```python
from build123d import *

# Parameters (mm, degrees)
BOSS_EXTRUDE1_DEPTH     = 12.5
SKETCH3_W               = 25
SKETCH3_H               = 11.5
CUT_EXTRUDE2_DEPTH      = 60.634302209
CUT_EXTRUDE1_DEPTH      = 60.634302209
CUT_EXTRUDE1_DEPTH_BACK = 60.634302209
SKETCH2_W               = 20.25
SKETCH2_H               = 8.5
SKETCH4_W               = 7.5
SKETCH4_H               = 20
CUT_EXTRUDE3_DEPTH      = 60.634302209
SKETCH8_R               = 2.55
PIN_HOLE_DEPTH          = 64.442887702
SKETCH9_R               = 3.5
COUNTERBORE_DEPTH       = 9
SKETCH7_R               = 2.55
CUT_EXTRUDE5_DEPTH      = 60.851900555
LPATTERN1_COUNT         = 2
LPATTERN1_PITCH         = 8.3
MIRROR2_COPY_1_SKETCH_R = 2.55
MIRROR2_COPY_1_DEPTH    = 60.851900555
FILLET1_R               = 5
CHAMFER1_SIZE           = 0.5
FILLET2_R               = 3


# Some blends are built 0.0001 mm under size
with BuildPart() as part:
    # Sketch1 → Boss-Extrude1 (new, symmetric)
    with BuildSketch(Plane.XY):
        Polygon((25, -30), (0, -30), (0, 30), (25, 30), (25, 0), (50, 0), (50, -30), align=None)
    extrude(amount=BOSS_EXTRUDE1_DEPTH, both=True)

    # Sketch3 → Cut-Extrude2 (cut, through all)
    with BuildSketch(Plane(origin=(0, 0, 0), x_dir=(1, 0, 0), z_dir=(0, 1, 0))):
        with Locations((37.5, -6.75)):
            Rectangle(SKETCH3_W, SKETCH3_H)
    extrude(amount=-CUT_EXTRUDE2_DEPTH, mode=Mode.SUBTRACT)

    # Sketch2 → Cut-Extrude1 (cut, two sides: drawn at the far end of the back side and taken through both)
    with BuildSketch(Plane(origin=(0, 0, 0), x_dir=(1, 0, 0), z_dir=(0, 1, 0)).offset(-CUT_EXTRUDE1_DEPTH_BACK)):
        with Locations((10.125, -5.25)):
            Rectangle(SKETCH2_W, SKETCH2_H)
    extrude(amount=CUT_EXTRUDE1_DEPTH + CUT_EXTRUDE1_DEPTH_BACK, mode=Mode.SUBTRACT)

    # Sketch4 → Cut-Extrude3 (cut, through all)
    with BuildSketch(Plane(origin=(50, 0, 0), x_dir=(0, 0, -1), z_dir=(1, 0, 0))):
        with Locations((5.75, -15)):
            Rectangle(SKETCH4_W, SKETCH4_H)
    extrude(amount=-CUT_EXTRUDE3_DEPTH, mode=Mode.SUBTRACT)

    # Mirror1: part across plane


with BuildPart() as part_1:
    add(part.part)
    add(part.part.mirror(Plane(origin=(0, 0, 0), x_dir=(0, 0, 1), z_dir=(1, 0, 0))))

    # Sketch8 → Pin Hole (cut, through all)
    with BuildSketch(Plane.XY.offset(12.5)):
        with Locations((0, 22.5)):
            Circle(SKETCH8_R)
        with Locations((0, 2.5)):
            Circle(SKETCH8_R)
    extrude(amount=-PIN_HOLE_DEPTH, mode=Mode.SUBTRACT)

    # Sketch9 → Counterbore (cut)
    with BuildSketch(Plane(origin=(0, 0, -12.5), x_dir=(-1, 0, 0), z_dir=(0, 0, -1))):
        with Locations((0, 22.5)):
            Circle(SKETCH9_R)
        with Locations((0, 2.5)):
            Circle(SKETCH9_R)
    extrude(amount=-COUNTERBORE_DEPTH, mode=Mode.SUBTRACT)

    # Sketch7 → Cut-Extrude5 (cut, through all)
    with BuildSketch(Plane.XY.offset(1)):
        with Locations((42.5, -15)):
            Circle(SKETCH7_R)
    cut_extrude5 = extrude(amount=-CUT_EXTRUDE5_DEPTH, mode=Mode.SUBTRACT)

    # LPattern1: Cut-Extrude5 ×2
    with Locations(*[(-i * LPATTERN1_PITCH, 0, 0) for i in range(1, LPATTERN1_COUNT)]):
        add(cut_extrude5, mode=Mode.SUBTRACT)

    # Mirror2: Cut-Extrude5 across plane
    add(cut_extrude5.mirror(Plane(origin=(0, 0, 0), x_dir=(0, 0, 1), z_dir=(1, 0, 0))), mode=Mode.SUBTRACT)

    # Mirror2 copy 1 sketch → Mirror2 copy 1 (cut, through all)
    with BuildSketch(Plane(origin=(8.3, 0, 1), x_dir=(-1, 0, 0), z_dir=(0, 0, 1))):
        with Locations((42.5, 15)):
            Circle(MIRROR2_COPY_1_SKETCH_R)
    extrude(amount=-MIRROR2_COPY_1_DEPTH, mode=Mode.SUBTRACT)

    # Fillet1
    # the kernel refuses this fillet: 5 mm, written as the material it adds along each edge
    with BuildSketch(Plane(origin=(-25, 0, 1), x_dir=(0, 1, 0), z_dir=(0, 0, -1))) as fillet1_piece_1:
        with BuildLine():
            CenterArc((FILLET1_R, -FILLET1_R), FILLET1_R, 90, 90)
            Line((0, -FILLET1_R), (0, 0))
            Line((0, 0), (FILLET1_R, 0))
        make_face()
    extrude(amount=13.5)
    with BuildSketch(Plane(origin=(25, 0, 1), x_dir=(0, 1, 0), z_dir=(0, 0, -1))) as fillet1_piece_2:
        with BuildLine():
            CenterArc((FILLET1_R, FILLET1_R), FILLET1_R, 180, 90)
            Line((0, FILLET1_R), (0, 0))
            Line((0, 0), (FILLET1_R, 0))
        make_face()
    extrude(amount=13.5)
    # the kernel refuses this fillet: 5 mm, written as the material it takes off along each edge
    with BuildSketch(Plane(origin=(25, 30, 25), x_dir=(0, -1, 0), z_dir=(0, 0, -1)), Plane(origin=(-25, 30, 25), x_dir=(1, 0, 0), z_dir=(0, 0, -1))) as fillet1_2_piece_1:
        with BuildLine():
            CenterArc((FILLET1_R, FILLET1_R), FILLET1_R, 180, 90)
            Line((0, FILLET1_R), (0, 0))
            Line((0, 0), (FILLET1_R, 0))
        make_face()
    extrude(amount=50, mode=Mode.SUBTRACT)
    with BuildSketch(Plane(origin=(-50, 0, -25), x_dir=(1, 0, 0), z_dir=(0, 0, 1)), Plane(origin=(50, 0, -25), x_dir=(0, -1, 0), z_dir=(0, 0, 1)), Plane(origin=(50, -30, -25), x_dir=(-1, 0, 0), z_dir=(0, 0, 1))) as fillet1_2_piece_2:
        with BuildLine():
            CenterArc((FILLET1_R, -FILLET1_R), FILLET1_R, 90, 90)
            Line((0, -FILLET1_R), (0, 0))
            Line((0, 0), (FILLET1_R, 0))
        make_face()
    extrude(amount=38.5, mode=Mode.SUBTRACT)
    with BuildSketch(Plane(origin=(-50, -30, -25), x_dir=(1, 0, 0), z_dir=(0, 0, 1))) as fillet1_2_piece_3:
        with BuildLine():
            CenterArc((FILLET1_R, FILLET1_R), FILLET1_R, 180, 90)
            Line((0, FILLET1_R), (0, 0))
            Line((0, 0), (FILLET1_R, 0))
        make_face()
    extrude(amount=38.5, mode=Mode.SUBTRACT)

    # Chamfer1
    chamfer1_edges = [part_1.edges().sort_by_distance(p)[0] for p in [
        (3.5, 22.5, -12.5),
        (3.5, 2.5, -12.5),
        (39.95, -15, -12.5),
        (31.65, -15, -12.5),
        (-39.95, -15, -12.5),
        (-31.65, -15, -12.5),
        (0, -30, -12.5),
        (-50, -15, -12.5),
        (-37.5, 0, -12.5),
        (-25, 15, -12.5),
        (0, 30, -12.5),
        (25, 15, -12.5),
        (37.5, 0, -12.5),
        (50, -15, -12.5),
        (48.535533906, -1.464466094, -12.5),
        (-48.535533906, -1.464466094, -12.5),
        (-23.535533906, 28.535533906, -12.5),
        (23.535533906, 28.535533906, -12.5),
        (48.535533906, -28.535533906, -12.5),
        (-48.535533906, -28.535533906, -12.5),
        (-26.464466094, 1.464466094, -12.5),
        (26.464466094, 1.464466094, -12.5),
    ]]
    chamfer(chamfer1_edges, length=CHAMFER1_SIZE)

    # Fillet2
    fillet2_edges = [part_1.edges().sort_by_distance(p)[0] for p in [
        (0, 30, 12.5),
        (-23.535533906, 28.535533906, 12.5),
        (23.535533906, 28.535533906, 12.5),
        (25, -2.5, 12.5),
        (25, -12.5, 1),
        (-25, -2.5, 12.5),
        (-25, -12.5, 1),
    ]]
    fillet(fillet2_edges, radius=FILLET2_R - 0.0001)  # a hair under: the kernel refuses the full size


solid = part_1.part
```
Check sheet for the modelled part. Datum: model origin and axes. Units: mm. A direction names the side the tool comes from. Round coordinates to 2 decimals unless told otherwise and drop trailing zeros. Order: outer loops, then holes, each group sorted by start corner. A loop starts at its lowest first (then second) coordinate and runs counter-clockwise, first axis right, second up. Notation, with made-up numbers: (-20.75, 22) -> (14.25, 22) arc R21 ccw to (14.25, 46) -> close; hole circle Ø4 at (44.5, 17). An arc over 180 degrees is marked (long way). One line per item, written item: value. Start each with the question number.
Q1. Set-up check for faces 5 (the face through (-2, 0, -3.5)), 6 (the face through (37, 0, -5)), 7 (the face through (25, 10, 1)): record each of +Z, -Z, +X, -X, +Y, -Y from which the full face is reachable in a straight line by a thin tool's end or side.
Q2. Cross-section at A-A (x = 17.5). Give the number of separate pieces and of enclosed holes in the cut face, and give its area (3 significant figures).
Q3. Cross-section at D-D (y = -6). Record the boundary of the cut face in (x, z), and give its area (4 significant figures).
Q4. Gauge pin test, flat ends, axial feed: pin 1 Ø11 at (x, y) = (0, 2.5) entering from -Z; pin 2 Ø11 at (x, y) = (44.5, -16) entering from +Z; pin 3 Ø4 at (x, y) = (0, 2.5) entering from +Z; pin 4 Ø10 at (y, z) = (23.5, 3) entering from +X. Record the tip position at first contact, or that the pin passes through.
Q5. Cross-section at B-B (y = 22.5). Record the boundary of the cut face in (x, z), and give its area (3 significant figures).
Q6. Cross-section at C-C (z = -6.25). Record the boundary of the cut face in (x, y).
Q7. Thickness scan on line 1 (Z direction, x = -7, y = -6); line 2 (Y direction, x = 42.5, z = -0.2); line 3 (Z direction, x = 43.5, y = -5.5). Record the ranges inside material, lowest first.
Q8. Mould release check, pull along Y, two halves, no side actions. Record for faces 1 (the face through (-48, -1, -6)), 2 (the face through (-39.952, -14.888, -10.732)), 3 (the face through (-0.33, 25.03, 11.02)), 4 (the face through (0.3, -0.4, 1)): pulls with the +Y half, pulls with the -Y half, needs draft (parallel to the pull), parting line crosses it, or undercut.
Completed:
1. face 5: -Z
1. face 6: +Z, -Z, +X, +Y
1. face 7: +Z, +X, +Y
2. separate pieces: 2
2. enclosed holes: 1
2. area: 838 mm²
3. outline: (-50, -12) -> (-49.5, -12.5) -> (49.5, -12.5) -> (50, -12) -> (50, -9.5) -> (-50, -9.5) -> close; (-50, -2) -> (50, -2) -> (50, 1) -> (28, 1) arc R3 cw to (25, 4) -> (25, 9.5) arc R3 ccw to (22, 12.5) -> (-22, 12.5) arc R3 ccw to (-25, 9.5) -> (-25, 4) arc R3 cw to (-28, 1) -> (-50, 1) -> close; hole (-20.25, 1) -> (20.25, 1) -> (20.25, 9.5) -> (-20.25, 9.5) -> close
3. area: 830.5 mm²
4. pin 1: stops at z = -12.5
4. pin 2: stops at z = 1
4. pin 3: passes through
4. pin 4: stops at x = 25
5. outline: (-25, -12) -> (-24.5, -12.5) -> (-4, -12.5) -> (-3.5, -12) -> (-3.5, -3.5) -> (-2.55, -3.5) -> (-2.55, 1) -> (-20.25, 1) -> (-20.25, 9.5) -> (-2.55, 9.5) -> (-2.55, 12.5) -> (-22, 12.5) arc R3 ccw to (-25, 9.5) -> close; (2.55, -3.5) -> (3.5, -3.5) -> (3.5, -12) -> (4, -12.5) -> (24.5, -12.5) -> (25, -12) -> (25, 9.5) arc R3 ccw to (22, 12.5) -> (2.55, 12.5) -> (2.55, 9.5) -> (20.25, 9.5) -> (20.25, 1) -> (2.55, 1) -> close
5. area: 800 mm²
6. outline: (-50, -25) arc R5 ccw to (-45, -30) -> (45, -30) arc R5 ccw to (50, -25) -> close; (-50, -5) -> (50, -5) arc R5 ccw to (45, 0) -> (30, 0) arc R5 cw to (25, 5) -> (25, 25) arc R5 ccw to (20, 30) -> (-20, 30) arc R5 ccw to (-25, 25) -> (-25, 5) arc R5 cw to (-30, 0) -> (-45, 0) arc R5 ccw to start; hole circle Ø7 at (0, 2.5); hole circle Ø7 at (0, 22.5)
7. line 1: z = -12.5 to -9.5, -2 to 1, 9.5 to 12.5
7. line 2: y = -30 to -17.55, -12.45 to 0
7. line 3: z = -12.5 to -9.5, -2 to 1
8. face 1: pulls with the +Y half
8. face 2: undercut
8. face 3: undercut
8. face 4: needs draft
